```python
from build123d import *

# Parameters (mm, degrees)
SKETCH1_W           = 95.25
SKETCH1_H           = 95.25
BOSS_EXTRUDE1_DEPTH = 38.1
SHELL1_T            = -6.35
BOSS_EXTRUDE2_DEPTH = 31.75
SKETCH3_R           = 1.905
SKETCH3_R_2         = 1.016
BOSS_EXTRUDE3_DEPTH = 6.35
SKETCH4_R           = 1.016
BOSS_EXTRUDE4_DEPTH = 8.89
SKETCH5_R           = 1.905
SKETCH5_W           = 24.1935
SKETCH5_H           = 5.08
BOSS_EXTRUDE5_DEPTH = 6.35
SKETCH7_R           = 1.016
BOSS_EXTRUDE6_DEPTH = 8.89
SKETCH8_R           = 2.38125
CUT_EXTRUDE1_DEPTH  = 8.89
BOSS_EXTRUDE7_DEPTH = 6.35
SKETCH12_W          = 10.16
SKETCH12_H          = 13.97
CUT_EXTRUDE2_DEPTH  = 6.35


with BuildPart() as part:
    # Sketch1 → Boss-Extrude1 (new body)
    with BuildSketch(Plane.XY):
        Rectangle(SKETCH1_W, SKETCH1_H)
    extrude(amount=BOSS_EXTRUDE1_DEPTH)

    # Shell1
    shell1_openings = [part.faces().sort_by_distance(p)[0] for p in [
        (0, 0, 38.1),
    ]]
    offset(amount=SHELL1_T, openings=shell1_openings, kind=Kind.INTERSECTION)

    # Sketch2 → Boss-Extrude2 (add)
    with BuildSketch(Plane.XY.offset(38.1)):
        with BuildLine():
            Line((-41.275, 41.275), (-36.195, 41.275))
            ThreePointArc((-36.195, 41.275), (-37.682897552, 37.682897552), (-41.275, 36.195))
            Line((-41.275, 36.195), (-41.275, 41.275))
        make_face()
        with BuildLine():
            Line((36.195, 41.275), (41.275, 41.275))
            Line((41.275, 41.275), (41.275, 36.195))
            ThreePointArc((41.275, 36.195), (37.682897552, 37.682897552), (36.195, 41.275))
        make_face()
        with BuildLine():
            Line((41.275, -36.195), (41.275, -41.275))
            Line((41.275, -41.275), (36.195, -41.275))
            ThreePointArc((36.195, -41.275), (37.682897552, -37.682897552), (41.275, -36.195))
        make_face()
        with BuildLine():
            Line((-41.275, -36.195), (-41.275, -41.275))
            Line((-41.275, -41.275), (-36.195, -41.275))
            ThreePointArc((-36.195, -41.275), (-37.682897552, -37.682897552), (-41.275, -36.195))
        make_face()
    extrude(amount=-BOSS_EXTRUDE2_DEPTH)

    # Sketch3 → Boss-Extrude3 (add)
    with BuildSketch(Plane.XY.offset(6.35)):
        with Locations((35.015710728, 31.115)):
            Circle(SKETCH3_R)
        with Locations((-10.704289272, 31.115)):
            Circle(SKETCH3_R_2)
        with Locations((-10.704289272, 13.335)):
            Circle(SKETCH3_R)
        with Locations((35.015710728, 13.335)):
            Circle(SKETCH3_R)
    extrude(amount=BOSS_EXTRUDE3_DEPTH)

    # Sketch4 → Boss-Extrude4 (add)
    with BuildSketch(Plane.XY.offset(12.7)):
        with Locations((-10.704289272, 31.115)):
            Circle(SKETCH4_R)
        with Locations((-10.704289272, 13.335)):
            Circle(SKETCH4_R)
        with Locations((35.015710728, 31.115)):
            Circle(SKETCH4_R)
        with Locations((35.015710728, 13.335)):
            Circle(SKETCH4_R)
    extrude(amount=BOSS_EXTRUDE4_DEPTH)

    # Sketch5 → Boss-Extrude5 (add)
    with BuildSketch(Plane.XY.offset(6.35)):
        with Locations((13.2715, -32.385)):
            Circle(SKETCH5_R)
        with Locations((33.655, -32.385)):
            Circle(SKETCH5_R)
        with Locations((23.46325, -4.445)):
            Rectangle(SKETCH5_W, SKETCH5_H)
    extrude(amount=BOSS_EXTRUDE5_DEPTH)

    # Sketch7 → Boss-Extrude6 (add)
    with BuildSketch(Plane.XY.offset(12.7)):
        with Locations((13.2715, -32.385)):
            Circle(SKETCH7_R)
        with Locations((33.655, -32.385)):
            Circle(SKETCH7_R)
    extrude(amount=BOSS_EXTRUDE6_DEPTH)

    # Sketch8 → Cut-Extrude1 (cut)
    with BuildSketch(Plane.XY.offset(38.1)):
        with Locations((-41.275, 41.275)):
            Circle(SKETCH8_R)
        with Locations((41.275, 41.275)):
            Circle(SKETCH8_R)
        with Locations((41.275, -41.275)):
            Circle(SKETCH8_R)
        with Locations((-41.275, -41.275)):
            Circle(SKETCH8_R)
    extrude(amount=-CUT_EXTRUDE1_DEPTH, mode=Mode.SUBTRACT)

    # Sketch10 → Boss-Extrude7 (add)
    with BuildSketch(Plane.XY.offset(6.35)):
        Polygon((-37.696932409, -30.607), (-37.696932409, 2.9972), (-1.781332409, 2.9972), (-1.781332409, -30.607), (-6.861332409, -30.607), (-6.861332409, -2.0828), (-32.616932409, -2.0828), (-32.616932409, -30.607), align=None)
    extrude(amount=BOSS_EXTRUDE7_DEPTH)

    # Sketch12 → Cut-Extrude2 (cut)
    with BuildSketch(Plane(origin=(47.625, 0, 0), x_dir=(0, 0, -1), z_dir=(1, 0, 0))):
        with Locations((-15.24, 22.225)):
            Rectangle(SKETCH12_W, SKETCH12_H)
    extrude(amount=-CUT_EXTRUDE2_DEPTH, mode=Mode.SUBTRACT)


solid = part.part
```
Part model, mm, in its own coordinate system. A direction names the side the tool comes from. Give positions to 0.01 mm unless a question says otherwise; leave off trailing zeros. Loops run counter-clockwise (first coordinate to the right, second up) from the corner with the lowest first, then second, coordinate; pieces in that order, holes last. Notation, with made-up numbers: M 36,80 L 44,80 A23 ccw 44,102 Z; hole C -9.5,17.25 d6. An arc over 180 degrees is marked long. Return JSON: item names as keys, results as strings.
1) Saw through at C-C, the plane z = 32.5. List the corners of the cut face in (x, y) (1 decimal), then the cut area to 3 significant figures.
Calculated:
{"outline": "M -47.6,-47.6 L 47.6,-47.6 L 47.6,47.6 L -47.6,47.6 Z; hole C -41.3,-41.3 d4.8; hole C -41.3,41.3 d4.8; hole M -41.3,-36.2 A5.1 cw -36.2,-41.3 L 36.2,-41.3 A5.1 cw 41.3,-36.2 L 41.3,36.2 A5.1 cw 36.2,41.3 L -36.2,41.3 A5.1 cw -41.3,36.2 Z; hole C 41.3,-41.3 d4.8; hole C 41.3,41.3 d4.8", "area": "2,270 mm2"}
2) Pull direction Y, two halves, no side cores. Call faces 4 (the face through (-41.275, -1, 22)), 5 (the face through (34.5, -33.2, 12.7)), 6 (the face through (47.625, -1, 19)): released by +Y, released by -Y, zero draft, split by the parting line, or undercut.
Calculated:
{"face 4": "undercut", "face 5": "undercut", "face 6": "zero draft"}
3) Drill centre lines: line 1 (Y direction, x = 34.5, z = 36) (3 decimals); line 2 (Z direction, x = 42.5, y = 28.5). Where is each one in solid material? Low to high.
Calculated:
{"line 1": "y = -47.625 to -41.275, 41.275 to 47.625", "line 2": "z = 0 to 10.16, 20.32 to 38.1"}
4) Saw through at D-D, the plane x = 27. List the corners of the cut face in (y, z) (3 decimals), then the cut area to 3 significant figures.
Calculated:
{"outline": "M -47.625,0 L 47.625,0 L 47.625,38.1 L 41.275,38.1 L 41.275,6.35 L -1.905,6.35 L -1.905,12.7 L -6.985,12.7 L -6.985,6.35 L -41.275,6.35 L -41.275,38.1 L -47.625,38.1 Z", "area": "1,040 mm2"}
5) 3-axis set-ups, long thin cutter, end or side, ignore diameter. For faces 1 (the face through (-37.644, -37.723, 22.447)), 2 (the face through (-47.625, -1, 19)), 3 (the face through (44, 22, 20.32)): which of +Z, -Z, +X, -X, +Y, -Y reach the whole face in a straight line?
Calculated:
{"face 1": "+Z", "face 2": "+Z, -Z, -X, +Y, -Y", "face 3": "+X"}
6) Flat gauge pins, fed straight in: pin 1 Ø1 at (x, y) = (33.5, -32.5) entering from +Z; pin 2 Ø10 at (x, y) = (-18, -15.5) entering from +Z; pin 3 Ø6 at (x, y) = (13, 4) entering from -Z; pin 4 Ø5.5 at (x, y) = (27, -3) entering from +Z. Where does each tip first touch, or does it go through?
Calculated:
{"pin 1": "stops at z = 21.59", "pin 2": "stops at z = 6.35", "pin 3": "stops at z = 0", "pin 4": "stops at z = 12.7"}
7) Saw through at B-B, the plane z = 24. List the corners of the cut face in (x, y) (3 decimals), then the cut area to 3 significant figures.
Calculated:
{"outline": "M -47.625,-47.625 L 47.625,-47.625 L 47.625,47.625 L -47.625,47.625 Z; hole M -41.275,-36.195 A5.08 cw -36.195,-41.275 L 36.195,-41.275 A5.08 cw 41.275,-36.195 L 41.275,36.195 A5.08 cw 36.195,41.275 L -36.195,41.275 A5.08 cw -41.275,36.195 Z", "area": "2,340 mm2"}
8) Saw through at A-A, the plane y = 20.5. List the corners of the cut face in (x, z) (3 decimals), then the cut area to 3 significant figures.
Calculated:
{"outline": "M -47.625,0 L 47.625,0 L 47.625,10.16 L 41.275,10.16 L 41.275,6.35 L -41.275,6.35 L -41.275,38.1 L -47.625,38.1 Z; M 41.275,20.32 L 47.625,20.32 L 47.625,38.1 L 41.275,38.1 Z", "area": "944 mm2"}
